Here's how the part is built. I have some questions about the finished solid (model axes, mm). Face numbers are marked on the shaded views. A direction names the side the tool comes from. Give positions to 0.01 mm unless a question says otherwise; leave off trailing zeros. Loops run counter-clockwise (first coordinate to the right, second up) from the corner with the lowest first, then second, coordinate; pieces in that order, holes last. Notation, with made-up numbers: (-15, -15) - (37, -15) arc R21 ccw to (37, -1) - close; hole circle Ø11 at (1.5, 5.25). An arc over 180 degrees is marked (long way). Return JSON: item names as keys, results as strings. Group by question number.
(1) On a 3-axis mill with a long thin cutter (end or side, diameter ignored), from which of +Z, -Z, +X, -X, +Y, -Y can I reach the whole of each face in a straight line? I mean the marked faces 4 and 5. Say none if no direction works.
(2) I need wall thicknesses on probe 1 along Z at (x, y) = (0, 0.9); probe 2 along Z at (x, y) = (-17, -0.5); probe 3 along Z at (x, y) = (-16, 2.5). Which ranges of each line are inside material? Lowest first, please. Write a range as [from, to].
(3) If we section it at C-C (z = 22): Please give me the cut outline in (x, y).
(4) If we section it at B-B (y = 2.75): State how many separate pieces and enclosed holes the cut face has, then the cut area to 3 significant figures.
(5) If we section it at A-A (x = 21): Please give me the cut outline in (y, z), then the cut area to 3 significant figures.
(6) If we mould it in two halves opening along X, with no side actions, what happens to the marked faces 1, 2 and 3? For each: released by +X, released by -X, zero draft, split by the parting line, or undercut.
(7) For P1, Ø1.5, axis at y = -3, z = 13, coming from the -X side; P2, Ø3, axis at x = 18.5, y = -2.5, coming from the -Z side; P3, Ø1.5, axis at y = -0.5, z = 9, coming from the -X side, each with a flat end and sliding along its axis, tell me the tip position at first contact or that it passes through.
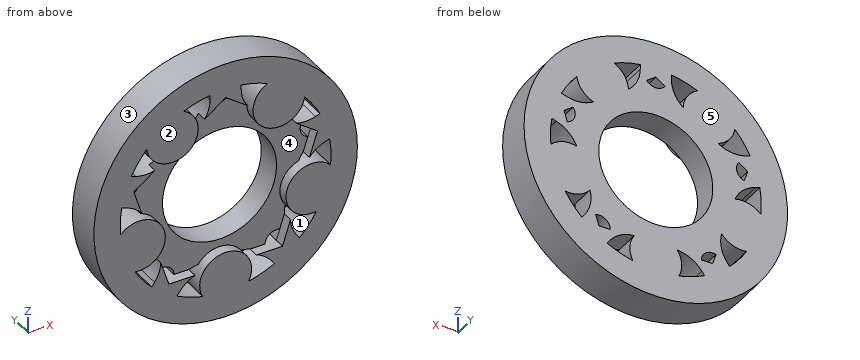
```python
from build123d import *

# Parameters (mm, degrees)
F0_R     = 25.4
F0_R_2   = 11
F1_DEPTH = 3.5
F2_R     = 11
F3_DEPTH = 2
F5_DEPTH = 25.4
F6_R     = 5.0054287193
F7_DEPTH = 7


with BuildPart() as f1:
    # F0 (on Front) → F1 (new body, symmetric)
    with BuildSketch(Plane.XZ):
        Circle(F0_R)
        with BuildLine():
            ThreePointArc((9.3858592072, -18.022431771), (0, -20.32), (-9.3858592072, -18.022431771))
            Line((-9.3858592072, -18.022431771), (-8.8547516049, -17.2914248694))
            ThreePointArc((-8.8547516049, -17.2914248694), (-6.0948306116, -15.1356722669), (-2.6118222651, -14.7708626849))
            ThreePointArc((-2.6118222651, -14.7708626849), (0, -15), (2.6118222651, -14.7708626849))
            ThreePointArc((2.6118222651, -14.7708626849), (6.0948306116, -15.1356722669), (8.8547516049, -17.2914248694))
            Line((8.8547516049, -17.2914248694), (9.3858592072, -18.022431771))
        make_face(mode=Mode.SUBTRACT)
        with BuildLine():
            ThreePointArc((-14.2399611735, -14.4957202573), (-19.3254684111, -6.2792253257), (-20.0407411772, 3.3572448629))
            Line((-20.0407411772, 3.3572448629), (-19.181391025, 3.0780250724))
            ThreePointArc((-19.181391025, 3.0780250724), (-16.2782859748, 1.1193484171), (-14.855022674, -2.0804570066))
            ThreePointArc((-14.855022674, -2.0804570066), (-14.2658477444, -4.6352549156), (-13.2408277416, -7.0484381758))
            ThreePointArc((-13.2408277416, -7.0484381758), (-12.5114735012, -10.4737083206), (-13.7088535712, -13.7647133557))
            Line((-13.7088535712, -13.7647133557), (-14.2399611735, -14.4957202573))
        make_face(mode=Mode.SUBTRACT)
        Circle(F0_R_2, mode=Mode.SUBTRACT)
        with BuildLine():
            ThreePointArc((20.0407411772, 3.3572448629), (19.3254684111, -6.2792253257), (14.2399611735, -14.4957202573))
            Line((14.2399611735, -14.4957202573), (13.7088535712, -13.7647133557))
            ThreePointArc((13.7088535712, -13.7647133557), (12.5114735012, -10.4737083206), (13.2408277416, -7.0484381758))
            ThreePointArc((13.2408277416, -7.0484381758), (14.2658477444, -4.6352549156), (14.855022674, -2.0804570066))
            ThreePointArc((14.855022674, -2.0804570066), (16.2782859748, 1.1193484171), (19.181391025, 3.0780250724))
            Line((19.181391025, 3.0780250724), (20.0407411772, 3.3572448629))
        make_face(mode=Mode.SUBTRACT)
        with BuildLine():
            ThreePointArc((-18.1866392109, 9.0635839606), (-11.9437963266, 16.4392253257), (-3, 20.0973232048))
            Line((-3, 20.0973232048), (-3, 19.1937489824))
            ThreePointArc((-3, 19.1937489824), (-3.9657033994, 15.8274676339), (-6.5690866511, 13.4850695427))
            ThreePointArc((-6.5690866511, 13.4850695427), (-8.8167787844, 12.1352549156), (-10.7951038486, 10.4146883246))
            ThreePointArc((-10.7951038486, 10.4146883246), (-13.8273464846, 8.6625645365), (-17.3272890587, 8.7843641702))
            Line((-17.3272890587, 8.7843641702), (-18.1866392109, 9.0635839606))
        make_face(mode=Mode.SUBTRACT)
        with BuildLine():
            Line((3, 19.1937489824), (3, 20.0973232048))
            ThreePointArc((3, 20.0973232048), (11.9437963266, 16.4392253257), (18.1866392109, 9.0635839606))
            Line((18.1866392109, 9.0635839606), (17.3272890587, 8.7843641702))
            ThreePointArc((17.3272890587, 8.7843641702), (13.8273464846, 8.6625645365), (10.7951038486, 10.4146883246))
            ThreePointArc((10.7951038486, 10.4146883246), (8.8167787844, 12.1352549156), (6.5690866511, 13.4850695427))
            ThreePointArc((6.5690866511, 13.4850695427), (3.9657033994, 15.8274676339), (3, 19.1937489824))
        make_face(mode=Mode.SUBTRACT)
    extrude(amount=F1_DEPTH, both=True)

    # F2 (on face) → F3 (cut)
    with BuildSketch(Plane.XZ.offset(3.5)):
        with BuildLine():
            Line((5.9151542337, -15.0662788144), (10.9462922974, -15.0662788144))
            Line((10.9462922974, -15.0662788144), (12.5009994602, -10.2813821745))
            ThreePointArc((12.5009994602, -10.2813821745), (12.6561218663, -8.6157571432), (13.2408277416, -7.0484381758))
            ThreePointArc((13.2408277416, -7.0484381758), (14.2658477444, -4.6352549156), (14.855022674, -2.0804570066))
            ThreePointArc((14.855022674, -2.0804570066), (15.3032326588, -0.468787836), (16.1567658253, 0.9699097832))
            Line((16.1567658253, 0.9699097832), (17.711472988, 5.7548064231))
            Line((17.711472988, 5.7548064231), (13.6411967935, 8.7120351792))
            ThreePointArc((13.6411967935, 8.7120351792), (12.1050287134, 9.3742717954), (10.7951038486, 10.4146883246))
            ThreePointArc((10.7951038486, 10.4146883246), (8.8167787844, 12.1352549156), (6.5690866511, 13.4850695427))
            ThreePointArc((6.5690866511, 13.4850695427), (5.1748026867, 14.4093757325), (4.0702761946, 15.6657160264))
            Line((4.0702761946, 15.6657160264), (0, 18.6229447825))
            Line((0, 18.6229447825), (-4.0702761946, 15.6657160264))
            ThreePointArc((-4.0702761946, 15.6657160264), (-5.1748026867, 14.4093757325), (-6.5690866511, 13.4850695427))
            ThreePointArc((-6.5690866511, 13.4850695427), (-8.8167787844, 12.1352549156), (-10.7951038486, 10.4146883246))
            ThreePointArc((-10.7951038486, 10.4146883246), (-12.1050287134, 9.3742717954), (-13.6411967935, 8.7120351792))
            Line((-13.6411967935, 8.7120351792), (-17.711472988, 5.7548064231))
            Line((-17.711472988, 5.7548064231), (-16.1567658253, 0.9699097832))
            ThreePointArc((-16.1567658253, 0.9699097832), (-15.3032326588, -0.468787836), (-14.855022674, -2.0804570066))
            ThreePointArc((-14.855022674, -2.0804570066), (-14.2658477444, -4.6352549156), (-13.2408277416, -7.0484381758))
            ThreePointArc((-13.2408277416, -7.0484381758), (-12.6561218663, -8.6157571432), (-12.5009994602, -10.2813821745))
            Line((-12.5009994602, -10.2813821745), (-10.9462922974, -15.0662788144))
            Line((-10.9462922974, -15.0662788144), (-5.9151542337, -15.0662788144))
            ThreePointArc((-5.9151542337, -15.0662788144), (-4.2831152343, -14.6991025487), (-2.6118222651, -14.7708626849))
            ThreePointArc((-2.6118222651, -14.7708626849), (0, -15), (2.6118222651, -14.7708626849))
            ThreePointArc((2.6118222651, -14.7708626849), (4.2831152343, -14.6991025487), (5.9151542337, -15.0662788144))
        make_face()
        Circle(F2_R, mode=Mode.SUBTRACT)
    extrude(amount=-F3_DEPTH, mode=Mode.SUBTRACT)

    # F4 (on face) → F5 (cut)
    with BuildSketch(Plane.XZ.offset(1.5)):
        with BuildLine():
            ThreePointArc((-15.5496324927, 5.7548064231), (-15.6554404977, 6.4228518753), (-15.9625072881, 7.0255043841))
            Line((-15.9625072881, 7.0255043841), (-17.711472988, 5.7548064231))
            Line((-17.711472988, 5.7548064231), (-17.0434275358, 3.6987739328))
            ThreePointArc((-17.0434275358, 3.6987739328), (-15.9625072881, 4.4841084621), (-15.5496324927, 5.7548064231))
        make_face()
        with BuildLine():
            ThreePointArc((-8.7844518021, -15.0662788144), (-9.6755943364, -13.3173131145), (-11.6143377496, -13.0102463241))
            Line((-11.6143377496, -13.0102463241), (-10.9462922974, -15.0662788144))
            Line((-10.9462922974, -15.0662788144), (-8.7844518021, -15.0662788144))
        make_face()
        with BuildLine():
            Line((10.9462922974, -15.0662788144), (11.6143377496, -13.0102463241))
            ThreePointArc((11.6143377496, -13.0102463241), (9.6755943364, -13.3173131145), (8.7844518021, -15.0662788144))
            Line((8.7844518021, -15.0662788144), (10.9462922974, -15.0662788144))
        make_face()
        with BuildLine():
            Line((17.711472988, 5.7548064231), (15.9625072881, 7.0255043841))
            ThreePointArc((15.9625072881, 7.0255043841), (15.6554404977, 5.0867609709), (17.0434275358, 3.6987739328))
            Line((17.0434275358, 3.6987739328), (17.711472988, 5.7548064231))
        make_face()
        with BuildLine():
            Line((0, 18.6229447825), (-1.7489656999, 17.3522468215))
            ThreePointArc((-1.7489656999, 17.3522468215), (0, 16.4611042872), (1.7489656999, 17.3522468215))
            Line((1.7489656999, 17.3522468215), (0, 18.6229447825))
        make_face()
    extrude(amount=-F5_DEPTH, mode=Mode.SUBTRACT)

    # F6 (on face) → F7 (join)
    with BuildSketch(Plane.XZ.offset(3.5)):
        with Locations((-10.2844180941, 14.1552871273)):
            Circle(F6_R)
        with Locations((-16.6405380308, -5.4068385621)):
            Circle(F6_R)
        with Locations((0, -17.4968971303)):
            Circle(F6_R)
        with Locations((16.6405380308, -5.4068385621)):
            Circle(F6_R)
        with Locations((10.2844180941, 14.1552871273)):
            Circle(F6_R)
    extrude(amount=-F7_DEPTH)


solid = f1.part
```
Values:
{
 "1": {"face 4": "-Y", "face 5": "+Z, -Z, +X, -X, +Y"},
 "2": {"probe 1": "[-25.4, -11], [11, 16.46], [18.62, 25.4]", "probe 2": "[-18.87, -11.13], [-10.4, -0.41], [1.85, 3.71], [6.27, 8.69], [11.13, 18.87]", "probe 3": "[-19.73, -12.53], [-10.37, -0.44], [0.76, 4.43], [7, 8.51], [12.53, 19.73]"},
 "3": {"outline": "(-12.69, -3.5) - (12.69, -3.5) - (12.69, 3.5) - (-12.69, 3.5) - close"},
 "4": {"separate pieces": "1", "enclosed holes": "16", "area": "1,480 mm2"},
 "5": {"outline": "(-3.5, -14.29) - (3.5, -14.29) - (3.5, 14.29) - (-3.5, 14.29) - close", "area": "200 mm2"},
 "6": {"face 1": "undercut", "face 2": "zero draft", "face 3": "split by the parting line"},
 "7": {"P1": "x = -22.25", "P2": "z = -18.87", "P3": "x = -24.02"}
}
